Design review of the part built by this model. Coordinates are the model's own, in mm. Face numbers are marked on the shaded views. A direction names the side the tool comes from. Give positions to 0.01 mm unless a question says otherwise; leave off trailing zeros. Order: outer loops, then holes, each group sorted by start corner. A loop starts at its lowest first (then second) coordinate and runs counter-clockwise, first axis right, second up. Notation, with made-up numbers: M 31.25,66 L 83.25,66 A35 cw 83.25,98 Z; hole C 77,-8 d4. An arc over 180 degrees is marked long. Answer as a JSON object with one key per item and string values.
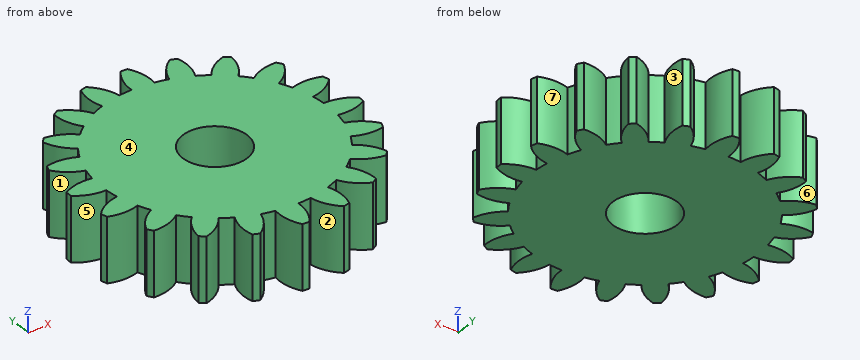
Autodesk Inventor part; units mm, degrees
ref_plane "YZ Plane" through (0, 0, 0) normal (1, 0, 0) x (0, 1, 0)
ref_plane "XZ Plane" through (0, 0, 0) normal (0, 1, 0) x (-1, 0, 0)
ref_plane "XY Plane" through (0, 0, 0) normal (0, 0, 1) x (1, 0, 0)
sketch "Sketch1" plane through (0, 0, 0) normal (0, 0, 1) x (1, 0, 0)
  arc A0 (21.8933, -2.1639) -> (21.9716, -1.1171) centre (0, 0) ccw
  circle A1 centre (0, 0) radius 17.5
  line L0 (0, 0) -> (28.7195, 0) construction
  arc A2 (21.9716, -1.1171) -> (17.4952, 0.4105) centre (17.6604, -6.4279) ccw
  line L1 (0, 0) -> (30.5019, 0) construction
  arc A3 (17.2394, -3.0086) -> (21.8933, -2.1639) centre (18.4202, 3.7291) ccw
  arc A4 (21.4905, 4.7074) -> (21.2414, 5.7272) centre (0, 0) ccw
  arc A5 (21.2414, 5.7272) -> (16.512, 5.7967) centre (18.7824, -0.6559) ccw
  arc A6 (17.3254, 2.4659) -> (21.4905, 4.7074) centre (16.3662, 9.2388) ccw
  arc A7 (18.984, 11.1179) -> (18.432, 12.0109) centre (0, 0) ccw
  arc A8 (18.432, 12.0109) -> (13.9126, 10.6155) centre (18.0658, 5.1803) ccw
  arc A9 (15.7154, 7.6991) -> (18.984, 11.1179) centre (12.7103, 13.844) ccw
  arc A10 (14.6192, 16.4401) -> (13.8183, 17.1188) centre (0, 0) ccw
  arc A11 (13.8183, 17.1188) -> (9.9513, 14.3952) centre (15.5808, 10.5094) ccw
  arc A12 (12.5671, 12.1786) -> (14.6192, 16.4401) centre (7.8102, 17.0942) ccw
  arc A13 (8.8234, 20.1531) -> (7.852, 20.5511) centre (0, 0) ccw
  arc A14 (7.852, 20.5511) -> (5.0159, 16.7658) centre (11.5707, 14.8098) ccw
  arc A15 (8.1886, 15.466) -> (8.8234, 20.1531) centre (2.1455, 18.671) ccw
  arc A16 (2.1639, 21.8933) -> (1.1171, 21.9716) centre (0, 0) ccw
  arc A17 (1.1171, 21.9716) -> (-0.4105, 17.4952) centre (6.4279, 17.6604) ccw
  arc A18 (3.0086, 17.2394) -> (2.1639, 21.8933) centre (-3.7291, 18.4202) ccw
  arc A19 (-4.7074, 21.4905) -> (-5.7272, 21.2414) centre (0, 0) ccw
  arc A20 (-5.7272, 21.2414) -> (-5.7967, 16.512) centre (0.6559, 18.7824) ccw
  arc A21 (-2.4659, 17.3254) -> (-4.7074, 21.4905) centre (-9.2388, 16.3662) ccw
  arc A22 (-11.1179, 18.984) -> (-12.0109, 18.432) centre (0, 0) ccw
  arc A23 (-12.0109, 18.432) -> (-10.6155, 13.9126) centre (-5.1803, 18.0658) ccw
  arc A24 (-7.6991, 15.7154) -> (-11.1179, 18.984) centre (-13.844, 12.7103) ccw
  arc A25 (-16.4401, 14.6192) -> (-17.1188, 13.8183) centre (0, 0) ccw
  arc A26 (-17.1188, 13.8183) -> (-14.3952, 9.9513) centre (-10.5094, 15.5808) ccw
  arc A27 (-12.1786, 12.5671) -> (-16.4401, 14.6192) centre (-17.0942, 7.8102) ccw
  arc A28 (-20.1531, 8.8234) -> (-20.5511, 7.852) centre (0, 0) ccw
  arc A29 (-20.5511, 7.852) -> (-16.7658, 5.0159) centre (-14.8098, 11.5707) ccw
  arc A30 (-15.466, 8.1886) -> (-20.1531, 8.8234) centre (-18.671, 2.1455) ccw
  arc A31 (-21.8933, 2.1639) -> (-21.9716, 1.1171) centre (0, 0) ccw
  arc A32 (-21.9716, 1.1171) -> (-17.4952, -0.4105) centre (-17.6604, 6.4279) ccw
  arc A33 (-17.2394, 3.0086) -> (-21.8933, 2.1639) centre (-18.4202, -3.7291) ccw
  arc A34 (-21.4905, -4.7074) -> (-21.2414, -5.7272) centre (0, 0) ccw
  arc A35 (-21.2414, -5.7272) -> (-16.512, -5.7967) centre (-18.7824, 0.6559) ccw
  arc A36 (-17.3254, -2.4659) -> (-21.4905, -4.7074) centre (-16.3662, -9.2388) ccw
  arc A37 (-18.984, -11.1179) -> (-18.432, -12.0109) centre (0, 0) ccw
  arc A38 (-18.432, -12.0109) -> (-13.9126, -10.6155) centre (-18.0658, -5.1803) ccw
  arc A39 (-15.7154, -7.6991) -> (-18.984, -11.1179) centre (-12.7103, -13.844) ccw
  arc A40 (-14.6192, -16.4401) -> (-13.8183, -17.1188) centre (0, 0) ccw
  arc A41 (-13.8183, -17.1188) -> (-9.9513, -14.3952) centre (-15.5808, -10.5094) ccw
  arc A42 (-12.5671, -12.1786) -> (-14.6192, -16.4401) centre (-7.8102, -17.0942) ccw
  arc A43 (-8.8234, -20.1531) -> (-7.852, -20.5511) centre (0, 0) ccw
  arc A44 (-7.852, -20.5511) -> (-5.0159, -16.7658) centre (-11.5707, -14.8098) ccw
  arc A45 (-8.1886, -15.466) -> (-8.8234, -20.1531) centre (-2.1455, -18.671) ccw
  arc A46 (-2.1639, -21.8933) -> (-1.1171, -21.9716) centre (0, 0) ccw
  arc A47 (-1.1171, -21.9716) -> (0.4105, -17.4952) centre (-6.4279, -17.6604) ccw
  arc A48 (-3.0086, -17.2394) -> (-2.1639, -21.8933) centre (3.7291, -18.4202) ccw
  arc A49 (4.7074, -21.4905) -> (5.7272, -21.2414) centre (0, 0) ccw
  arc A50 (5.7272, -21.2414) -> (5.7967, -16.512) centre (-0.6559, -18.7824) ccw
  arc A51 (2.4659, -17.3254) -> (4.7074, -21.4905) centre (9.2388, -16.3662) ccw
  arc A52 (11.1179, -18.984) -> (12.0109, -18.432) centre (0, 0) ccw
  arc A53 (12.0109, -18.432) -> (10.6155, -13.9126) centre (5.1803, -18.0658) ccw
  arc A54 (7.6991, -15.7154) -> (11.1179, -18.984) centre (13.844, -12.7103) ccw
  arc A55 (16.4401, -14.6192) -> (17.1188, -13.8183) centre (0, 0) ccw
  arc A56 (17.1188, -13.8183) -> (14.3952, -9.9513) centre (10.5094, -15.5808) ccw
  arc A57 (12.1786, -12.5671) -> (16.4401, -14.6192) centre (17.0942, -7.8102) ccw
  arc A58 (20.1531, -8.8234) -> (20.5511, -7.852) centre (0, 0) ccw
  arc A59 (20.5511, -7.852) -> (16.7658, -5.0159) centre (14.8098, -11.5707) ccw
  arc A60 (15.466, -8.1886) -> (20.1531, -8.8234) centre (18.671, -2.1455) ccw
  point P0 (16.7658, -5.0159)
  point P1 (17.2394, -3.0086)
  point P2 (17.3254, 2.4659)
  point P3 (16.512, 5.7967)
  point P4 (13.9126, 10.6155)
  point P5 (12.5671, 12.1786)
  point P6 (9.9513, 14.3952)
  point P7 (5.0159, 16.7658)
  point P8 (3.0086, 17.2394)
  point P9 (-0.4105, 17.4952)
  point P10 (-2.4659, 17.3254)
  point P11 (-5.7967, 16.512)
  point P12 (-10.6155, 13.9126)
  point P13 (-12.1786, 12.5671)
  point P14 (-14.3952, 9.9513)
  point P15 (-16.7658, 5.0159)
  point P16 (-17.2394, 3.0086)
  point P17 (-17.4952, -0.4105)
  point P18 (-17.3254, -2.4659)
  point P19 (-16.512, -5.7967)
  point P20 (-13.9126, -10.6155)
  point P21 (-12.5671, -12.1786)
  point P22 (-9.9513, -14.3952)
  point P23 (-8.1886, -15.466)
  point P24 (-3.0086, -17.2394)
  point P25 (0.4105, -17.4952)
  point P26 (2.4659, -17.3254)
  point P27 (5.7967, -16.512)
  point P28 (10.6155, -13.9126)
  point P29 (12.1786, -12.5671)
  point P30 (15.466, -8.1886)
  dimension "d13" = 35
  dimension "d12" = 44
  dimension "d18" = 360
extrude "Extrusion1" add sketch "Sketch1" along normal blind 10
sketch "Sketch2" plane through (0, 0, 10) normal (0, 0, 1) x (1, 0, 0)
  circle A0 centre (0, 0) radius 5
  dimension "d20" = 10
extrude "Extrusion2" cut sketch "Sketch2" against normal blind 10
properties part number "ENGRANAJE PARA RODILLO"
(1) To check wall thickness, follow L1, parallel to X at y = -18.5, z = 4.75; L2, parallel to X at y = 20, z = 6. State the ranges of each line that lie inside material, in increasing order. Write a range as from..to.
Checked values:
{"L1": "x = -8.98..-5.81, -3.11..0.36, 2.74..6.18, 10.2..11.91", "L2": "x = -6.08..-3.44, 0..2.93, 7.12..8.86"}
(2) We need section A-A (x = 4). Write out the cut boundary in (y, z).
Checked values:
{"outline": "M -20.76,0 L -3,0 L -3,10 L -20.76,10 Z; M 3,0 L 17.04,0 L 17.04,10 L 3,10 Z"}
(3) Insertion check: pin 1 (9 mm diameter, centred on x = 0, y = 0, fed in from +Z); pin 2 (4 mm diameter, centred on x = -2.5, z = 3.5, fed in from +Y); pin 3 (3 mm diameter, centred on y = -4, z = 2, fed in from -X); pin 4 (4 mm diameter, centred on x = 7, z = 4.5, fed in from +Y). Each pin has a flat end and moves straight along its axis. Give the tip position at first contact, or say it passes through.
Checked values:
{"pin 1": "passes through", "pin 2": "stops at y = 21.3", "pin 3": "stops at x = -21.49", "pin 4": "stops at y = 20.55"}
(4) Draft analysis for pull direction Y (two halves, no side actions). For the marked faces 4, 5, 6 and 7, state which applies: +Y half, -Y half, draft (parallel to the pull), parting line (faces both ways), or undercut.
Checked values:
{"face 4": "draft", "face 5": "undercut", "face 6": "+Y half", "face 7": "undercut"}
(5) Tool access review of the marked faces 1, 2 and 3: name each direction out of +Z, -Z, +X, -X, +Y, -Y from which nothing blocks a thin tool from reaching the whole face with its end or side.
Checked values:
{"face 1": "+Z, -Z, -X", "face 2": "+Z, -Z, -Y", "face 3": "+Z, -Z"}
